Work out the finished part from the listing and answer in its coordinate system (mm). A direction names the side the tool comes from. Coordinates: 2 decimals unless noted, no trailing zeros. Loops run counter-clockwise (first coordinate to the right, second up) from the corner with the lowest first, then second, coordinate; pieces in that order, holes last. Notation, with made-up numbers: (64, 40.25) -> (109, 40.25) arc R30 ccw to (109, 76.25) -> close; hole circle Ø6 at (12, 67). An arc over 180 degrees is marked (long way). One line per question, with ' | ' between items.
Autodesk Inventor part; units mm, degrees
ref_plane "YZ Plane" through (0, 0, 0) normal (1, 0, 0) x (0, 1, 0)
ref_plane "XZ Plane" through (0, 0, 0) normal (0, 1, 0) x (-1, 0, 0)
ref_plane "XY Plane" through (0, 0, 0) normal (0, 0, 1) x (1, 0, 0)
ref_plane "Work Plane1" through (0, 0, 0) normal (0, 0, 1) x (1, 0, 0)
sketch "Sketch1" plane through (0, 0, 0) normal (0, 0, 1) x (1, 0, 0)
  line L0 (-10, 0) -> (-10, 6)
  line L1 (-10, 6) -> (-34, 6)
  line L2 (-34, 0) -> (-34, 6)
  line L3 (-34, 0) -> (-10, 0)
  line L4 (-10, 21) -> (-10, 27)
  line L5 (-10, 27) -> (-34, 27)
  line L6 (-34, 21) -> (-34, 27)
  line L7 (-34, 21) -> (-10, 21)
  line L8 (0, 21) -> (0, 27)
  line L9 (0, 21) -> (24, 21)
  line L10 (24, 21) -> (24, 27)
  line L11 (24, 27) -> (0, 27)
  line L12 (0, 0) -> (0, 6)
  line L13 (0, 0) -> (24, 0)
  line L14 (24, 0) -> (24, 6)
  line L15 (24, 6) -> (0, 6)
  line L16 (24, 8.5) -> (30, 8.5)
  line L17 (30, 8.5) -> (30, -1.5)
  line L18 (24, -1.5) -> (30, -1.5)
  line L19 (24, -1.5) -> (24, 8.5)
  line L20 (24, 18.5) -> (30, 18.5)
  line L21 (24, 18.5) -> (24, 28.5)
  line L22 (24, 28.5) -> (30, 28.5)
  line L23 (30, 28.5) -> (30, 18.5)
  line L24 (10, -15.5) -> (20, -15.5)
  line L25 (24, -11.5) -> (24, -1.5)
  line L26 (24, 28.5) -> (24, 38.5)
  line L27 (20, 42.5) -> (10, 42.5)
  line L28 (-20, 42.5) -> (-30, 42.5)
  line L29 (-34, 38.5) -> (-34, 28.5)
  line L30 (-34, 8.5) -> (-34, 18.5)
  line L31 (-34, -11.5) -> (-34, -1.5)
  line L32 (-30, -15.5) -> (-20, -15.5)
  line L33 (-10, -15.5) -> (0, -15.5)
  line L34 (10, -15.5) -> (20, -15.5)
  line L35 (-34, -15.5) -> (24, -15.5)
  line L36 (24, -15.5) -> (24, 42.5)
  line L37 (24, 42.5) -> (-34, 42.5)
  line L38 (-34, 42.5) -> (-34, -15.5)
  line L39 (-34, 8.5) -> (-40, 8.5)
  line L40 (-34, 8.5) -> (-34, -1.5)
  line L41 (-34, -1.5) -> (-40, -1.5)
  line L42 (-40, -1.5) -> (-40, 8.5)
  line L43 (-34, 18.5) -> (-40, 18.5)
  line L44 (-40, 18.5) -> (-40, 28.5)
  line L45 (-34, 28.5) -> (-40, 28.5)
  line L46 (-34, 28.5) -> (-34, 18.5)
  line L47 (0, 27) -> (-10, 27)
  line L48 (-10, 21) -> (-10, 27)
  line L49 (-10, 21) -> (0, 21)
  line L50 (0, 21) -> (0, 27)
  line L51 (0, 6) -> (-10, 6)
  line L52 (-10, 0) -> (-10, 6)
  line L53 (-10, 0) -> (0, 0)
  line L54 (0, 0) -> (0, 6)
extrude "Plate1" add sketch "Sketch1" along normal blind 6 contours L3 L2 L1 L0 | L53 L13 L19 L25 L36 L35 L24 L33 L32 L38 L31 L3 | L1 L38 L30 L7 L49 L9 L21 L36 L19 L15 L51 | L38 L41 L42 L39 L2 | L12 L15 L14 L13 | L14 L19 L16 L17 L18 | L43 L44 L45 L38 L6 | L6 L5 L4 L7 | L21 L10 L22 L23 L20 | L38 L29 L37 L28 L27 L36 L26 L21 L11 L47 L5 | L9 L8 L11 L10
sketch "Sketch2" plane through (0, 0, 6) normal (0, 0, 1) x (1, 0, 0)
  line L0 (-10, 27) -> (0, 27)
  line L1 (0, 27) -> (0, 21)
  line L2 (0, 21) -> (-10, 21)
  line L3 (-10, 21) -> (-10, 27)
  line L4 (0, 0) -> (-10, 0)
  line L5 (-10, 0) -> (-10, 6)
  line L6 (-10, 6) -> (0, 6)
  line L7 (0, 6) -> (0, 0)
  line L8 (30, -1.5) -> (24, -1.5)
  line L9 (30, 8.5) -> (30, -1.5)
  line L10 (24, 8.5) -> (30, 8.5)
  line L11 (24, 18.5) -> (24, 8.5)
  line L12 (30, 18.5) -> (24, 18.5)
  line L13 (30, 28.5) -> (30, 18.5)
  line L14 (24, 28.5) -> (30, 28.5)
  line L15 (24, 42.5) -> (24, 28.5)
  line L16 (-34, 42.5) -> (24, 42.5)
  line L17 (-34, 28.5) -> (-34, 42.5)
  line L18 (-40, 28.5) -> (-34, 28.5)
  line L19 (-40, 18.5) -> (-40, 28.5)
  line L20 (-34, 18.5) -> (-40, 18.5)
  line L21 (-34, 8.5) -> (-34, 18.5)
  line L22 (-40, 8.5) -> (-34, 8.5)
  line L23 (-40, -1.5) -> (-40, 8.5)
  line L24 (-34, -1.5) -> (-40, -1.5)
  line L25 (-34, -15.5) -> (-34, -1.5)
  line L26 (24, -15.5) -> (-34, -15.5)
  line L27 (24, -1.5) -> (24, -15.5)
  circle A0 centre (-5, 13.5) radius 2.5
  point P0 (0, 0)
  point P1 (-5, 6)
  point P2 (-34, 13.5)
  dimension "d1" = 5
extrude "Cut1" cut sketch "Sketch2" against normal blind 6 contours A0
equation "\"d2\" = Thickness"
equation "\"d0\" = Thickness"
equation "\"BendRadius\" = Thickness"
equation "\"BendReliefWidth\" = Thickness"
equation "\"BendReliefDepth\" = 0.5 * Thickness"
equation "\"CornerReliefSize\" = 4 * Thickness"
equation "\"MinimumRemnant\" = 2 * Thickness"
equation "\"TransitionRadius\" = BendRadius"
equation "\"JacobiRadiusSize\" = BendRadius"
equation "\"GapSize\" = Thickness"
properties part number "joystick binnenkant" material "Wood (Birch)"
1) The mould has two halves that part along X. Classify faces 6 (the face through (-3.85, 11.28, 3.04)), 7 (the face through (-40, 23, 3)), 8 (the face through (-37, 8.5, 3)): released by +X, released by -X, zero draft, split by the parting line, or undercut.
Check values:
face 6: undercut | face 7: released by -X | face 8: zero draft
2) Find the intervals of material crossed by line 1 along Y through (x, z) = (-5, 4.5); line 2 along X through (y, z) = (26.5, 3.4); line 3 along X through (y, z) = (30, 0.8), in increasing order.
Check values:
line 1: y = -15.5 to 0, 6 to 11, 16 to 21, 27 to 42.5 | line 2: x = -40 to -10, 0 to 30 | line 3: x = -34 to 24
3) Find section A-A (y = 5). Write down the section's boundary in (x, z).
Check values:
outline: (-40, 0) -> (-10, 0) -> (-10, 6) -> (-40, 6) -> close; (0, 0) -> (30, 0) -> (30, 6) -> (0, 6) -> close
4) For faces 1 (the face through (-37, 28.5, 3)), 2 (the face through (24, 13, 3)), 3 (the face through (-5, 21, 3)), 4 (the face through (24, 35, 3)), 5 (the face through (27, -1.5, 3)), determine the directions among +Z, -Z, +X, -X, +Y, -Y from which every point of the face is accessible in a straight line to the end or side of a thin tool.
Check values:
face 1: +Z, -Z, -X, +Y | face 2: +Z, -Z, +X | face 3: +Z, -Z | face 4: +Z, -Z, +X, +Y | face 5: +Z, -Z, +X, -Y
5) Find section B-B (x = -5). Write down the section's boundary in (y, z), plus the area to 3 significant figures.
Check values:
outline: (-15.5, 0) -> (0, 0) -> (0, 6) -> (-15.5, 6) -> close; (6, 0) -> (11, 0) -> (11, 6) -> (6, 6) -> close; (16, 0) -> (21, 0) -> (21, 6) -> (16, 6) -> close; (27, 0) -> (42.5, 0) -> (42.5, 6) -> (27, 6) -> close | area: 246 mm^2
6) Find section D-D (y = 13.5). Write down the section's boundary in (x, z), plus the area to 3 significant figures.
Check values:
outline: (-34, 0) -> (-7.5, 0) -> (-7.5, 6) -> (-34, 6) -> close; (-2.5, 0) -> (24, 0) -> (24, 6) -> (-2.5, 6) -> close | area: 318 mm^2
7) Find section C-C (z = 2.8). State how many separate pieces and enclosed holes the cut face has, plus the area to 3 significant figures.
Check values:
separate pieces: 1 | enclosed holes: 3 | area: 3,460 mm^2
8) Flat-ended cylindrical pins translate along their axes: pin 1 (3 mm diameter, centred on y = 14.5, z = 2, fed in from -X); pin 2 (1.8 mm diameter, centred on x = 26, z = 2.5, fed in from -Y); pin 3 (3 mm diameter, centred on y = -11.5, z = 4, fed in from +X). Find the tip coordinate at first contact, or state that the pin passes through.
Check values:
pin 1: stops at x = -34 | pin 2: stops at y = -1.5 | pin 3: stops at x = 24
